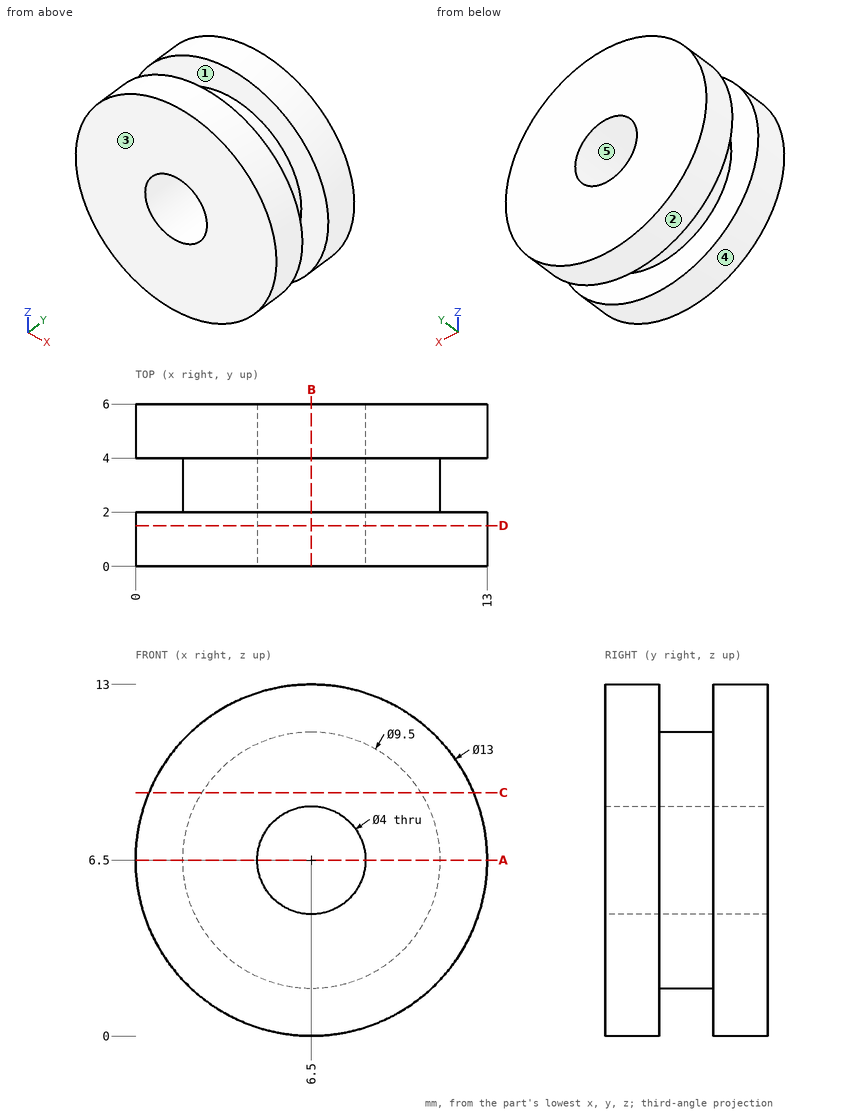
Job drawing, mm, ordinate dimensions from the low corner. One solid piece. A direction names the side the tool comes from. Give positions to 0.01 mm unless a question says otherwise; leave off trailing zeros. Loops run counter-clockwise (first coordinate to the right, second up) from the corner with the lowest first, then second, coordinate; pieces in that order, holes last. Notation, with made-up numbers: (49.25, 18) - (84.25, 18) arc R6 ccw to (84.25, 24) - close; hole circle Ø3 at (73.25, 26). An arc over 180 degrees is marked (long way). Use one line per item in the form item = value.
(1) Drop a flat-ended pin along its axis: P1, Ø1.5, axis at x = 5, y = 5, coming from the -Z side. Give the stop position or say it passes through.
Determined:
P1 = 0.04
(2) 3-axis set-ups, long thin cutter, end or side, ignore diameter. For the marked faces 1 and 2: which of +Z, -Z, +X, -X, +Y, -Y reach the whole face in a straight line?
Determined:
face_1 = none
face_2 = +Y, -Y
(3) Cut at D-D (y = 1.5). Give the cut face in (x, z).
Determined:
outline = circle Ø13 at (6.5, 6.5); hole circle Ø4 at (6.5, 6.5)
(4) Pull direction Z, two halves, no side cores. Call the marked faces 3, 4 and 5: pulls with the +Z half, pulls with the -Z half, needs draft (parallel to the pull), parting line crosses it, or undercut.
Determined:
face_3 = needs draft
face_4 = parting line crosses it
face_5 = undercut
(5) Drill centre lines: L1, parallel to X at y = 2.95, z = 6.5; L2, parallel to X at y = 1.9, z = 6.5; L3, parallel to Y at x = 1.25, z = 3. Where is each one in solid material? Low to high.
Determined:
L1 = 1.75 to 4.5, 8.5 to 11.25
L2 = 0 to 4.5, 8.5 to 13
L3 = 0 to 2, 4 to 6
(6) Cut at B-B (x = 6.5). Give the cut face in (y, z).
Determined:
outline = (0, 0) - (2, 0) - (2, 1.75) - (4, 1.75) - (4, 0) - (6, 0) - (6, 4.5) - (0, 4.5) - close; (0, 8.5) - (6, 8.5) - (6, 13) - (4, 13) - (4, 11.25) - (2, 11.25) - (2, 13) - (0, 13) - close
(7) Cut at A-A (z = 6.5). Give the cut face in (x, y).
Determined:
outline = (0, 0) - (4.5, 0) - (4.5, 6) - (0, 6) - (0, 4) - (1.75, 4) - (1.75, 2) - (0, 2) - close; (8.5, 0) - (13, 0) - (13, 2) - (11.25, 2) - (11.25, 4) - (13, 4) - (13, 6) - (8.5, 6) - close
(8) Cut at C-C (z = 9). Give the cut face in (x, y).
Determined:
outline = (0.5, 0) - (12.5, 0) - (12.5, 2) - (10.54, 2) - (10.54, 4) - (12.5, 4) - (12.5, 6) - (0.5, 6) - (0.5, 4) - (2.46, 4) - (2.46, 2) - (0.5, 2) - close
